Build history of the part. All positions in model axes, mm. Face numbers are marked on the shaded views. A direction names the side the tool comes from. Give positions to 0.01 mm unless a question says otherwise; leave off trailing zeros. Order: outer loops, then holes, each group sorted by start corner. A loop starts at its lowest first (then second) coordinate and runs counter-clockwise, first axis right, second up. Notation, with made-up numbers: (19, -27.5) -> (41, -27.5) arc R27 ccw to (41, -10.5) -> close; hole circle Ø6 at (-27, 0). An arc over 180 degrees is marked (long way). One line per item, written item: value. Start each with the question number.
(1) Two-plate mould, pull along X, no slides. Class the marked faces 1, 2, 3 and 4: +X half, -X half, draft (parallel to the pull), parting line (faces both ways), or undercut.
(2) Pin check, flat tips, straight feed: pin 1 (5 mm diameter, centred on y = 2.5, z = 16.5, fed in from -X); pin 2 (1 mm diameter, centred on x = -2.5, y = -15, fed in from +Z); pin 3 (8 mm diameter, centred on x = -10, y = -5, fed in from -Z). Stop position of each tip, or through.
(3) Probe line 1 (X direction, y = -17.5, z = -18.5); line 2 (Z direction, x = -0.5, y = 0); line 3 (X direction, y = 3, z = 22). List the from-to ranges inside material, lowest first.
(4) Saw through at A-A on z = 18. Give the cut face in (x, y), plus the area to 3 significant figures.
(5) Which spindle directions (+Z, -Z, +X, -X, +Y, -Y) get a long thin tool onto all of the face, cutting with end or side? Do the marked faces 5, 6, 7 and 8. Say none if no direction does.
(6) Saw through at D-D on x = -12. Give the cut face in (y, z), plus the area to 3 significant figures.
(7) Saw through at B-B on y = 0. Give the cut face in (x, z).
(8) Saw through at C-C on z = -9. Give the cut face in (x, y).
```python
from build123d import *

# Parameters (mm, degrees)
F1_DEPTH = 20
F3_DEPTH = 20
F5_D     = 2
F6_SIZE2 = 1.1547005384
F6_SIZE  = 2
F7_SIZE2 = 1.1547005384
F7_SIZE  = 2
F8_R     = 1
F9_R     = 2
F10_R    = 4
F11_R    = 8


with BuildPart() as f1:
    # F0 (on Front) → F1 (new body, symmetric)
    with BuildSketch(Plane.XZ):
        Polygon((0, 2), (0, 0), (0, -40), (2, -40), (2, 30), (0, 30), align=None)
        Polygon((-19.5, -40), (-19.5, 0), (0, 0), (0, 2), (-21.5, 2), (-21.5, -40), align=None)
    extrude(amount=F1_DEPTH, both=True)

    # F2 (on face) → F3 (join)
    with BuildSketch(Plane.XY.offset(30)):
        Polygon((0, -20), (0, 20), (-8, 6.1435935394), (-8, -6.1435935394), align=None)
    extrude(amount=-F3_DEPTH)

    # F5 (through all)
    with Locations(Plane.YZ.offset(2)):
        with Locations((0, 18)):
            Hole(F5_D / 2)

    # F6
    f6_edges = [f1.edges().sort_by_distance(p)[0] for p in [
        (-19.5, 0, -40),
    ]]
    f6_side = f1.faces().sort_by_distance((-19.5, 0, -20))[0]
    chamfer(f6_edges, length=F6_SIZE, length2=F6_SIZE2, reference=f6_side)

    # F7
    f7_edges = [f1.edges().sort_by_distance(p)[0] for p in [
        (0, 0, -40),
    ]]
    f7_side = f1.faces().sort_by_distance((0, 0, -20))[0]
    chamfer(f7_edges, length=F7_SIZE, length2=F7_SIZE2, reference=f7_side)

    # F8
    f8_edges = [f1.edges().sort_by_distance(p)[0] for p in [
        (-20.654701, 0, -40),
        (1.154701, 0, -40),
    ]]
    fillet(f8_edges, radius=F8_R)

    # F9
    f9_edges = [f1.edges().sort_by_distance(p)[0] for p in [
        (0, 0, 2),
        (-19.5, 0, 0),
        (0, 0, 0),
        (0, 0, 10),
    ]]
    fillet(f9_edges, radius=F9_R)

    # F10
    f10_edges = [f1.edges().sort_by_distance(p)[0] for p in [
        (-21.5, 0, 2),
        (-8, -6.143594, 20),
        (-8, 6.143594, 20),
        (-19.5, 0, -38),
        (0, 0, -38),
    ]]
    fillet(f10_edges, radius=F10_R)

    # F11
    f11_edges = [f1.edges().sort_by_distance(p)[0] for p in [
        (1, -20, 30),
        (1, 20, 30),
    ]]
    fillet(f11_edges, radius=F11_R)


solid = f1.part
```
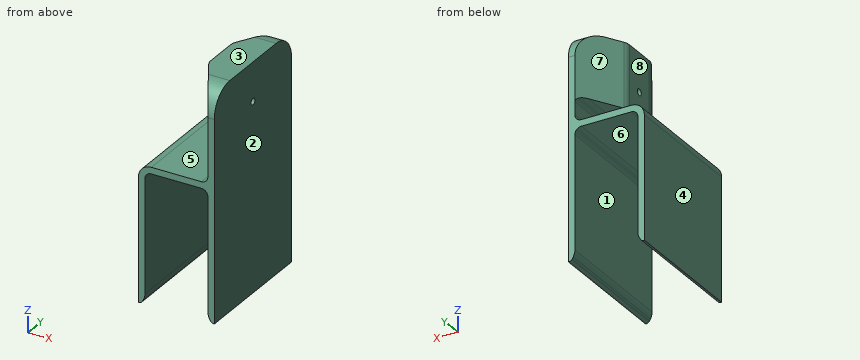
Results below:
1. face 1: undercut
1. face 2: +X half
1. face 3: draft
1. face 4: -X half
2. pin 1: stops at x = -8
2. pin 2: stops at z = 29.6
2. pin 3: stops at z = 0
3. line 1: x = -21.5 to -19.5, 0 to 2
3. line 2: z = -0.68 to 2.68, 9.32 to 17, 19 to 30
3. line 3: x = -8 to 2
4. outline: (-8, -5.07) arc R4 ccw to (-7.46, -7.07) -> (0, -20) -> (2, -20) -> (2, -1) -> (-8, -1) -> close; (-8, 1) -> (2, 1) -> (2, 20) -> (0, 20) -> (-7.46, 7.07) arc R4 ccw to (-8, 5.07) -> close
4. area: 269 mm²
5. face 5: -X, +Y, -Y
5. face 6: -Z, +Y, -Y
5. face 7: +Z, -X, +Y
5. face 8: +Z, -X, +Y, -Y
6. outline: (-20, 0) -> (20, 0) -> (20, 2) -> (-20, 2) -> close
6. area: 80.0 mm²
7. outline: (-21.5, -40) -> (-21.23, -40) arc R1 ccw to (-20.37, -39.5) -> (-20.04, -38.93) arc R4 ccw to (-19.5, -36.93) -> (-19.5, -2) arc R2 cw to (-17.5, 0) -> (-2, 0) arc R2 cw to (0, -2) -> (0, -36.93) arc R4 ccw to (0.54, -38.93) -> (0.87, -39.5) arc R1 ccw to (1.73, -40) -> (2, -40) -> (2, 17) -> (-8, 17) -> (-8, 10) -> (-2, 10) arc R2 cw to (0, 8) -> (0, 4) arc R2 cw to (-2, 2) -> (-17.5, 2) arc R4 ccw to (-21.5, -2) -> close; (-8, 19) -> (2, 19) -> (2, 30) -> (-8, 30) -> close
8. outline: (-21.5, -20) -> (-19.5, -20) -> (-19.5, 20) -> (-21.5, 20) -> close; (0, -20) -> (2, -20) -> (2, 20) -> (0, 20) -> close
